Here's how the part is built. I have some questions about the finished solid (model axes, mm). Face numbers are marked on the shaded views. Round coordinates to 2 decimals unless told otherwise and drop trailing zeros. Write each loop counter-clockwise with the first axis right and the second up, starting at its lowest first coordinate (ties: lowest second). Pieces come first, ordered by that corner, then holes. Notation, with made-up numbers: (-35.5, -20.5) - (16.5, -20.5) arc R15 ccw to (16.5, -16.5) - close; hole circle Ø6 at (21, 73.5). An arc over 180 degrees is marked (long way). One line per item, written item: value. Start each with the question number.
Item 1: Imagine slicing it at B-B, the plane y = -0.85. Please give me the cut outline in (x, z), then the cut area to 3 significant figures.
Item 2: Imagine slicing it at A-A, the plane z = -12. Please give me the cut outline in (x, y), then the cut area to 3 significant figures.
Item 3: If I drill on line 1 (X direction, y = -0.3, z = -4); line 2 (X direction, y = -2.65, z = 11), over which ranges is the centre line in solid material (lowest first)?
Item 4: Thinking about a two-plate mould opening in Y: for the marked faces 1 and 2, which applies, released by +Y, released by -Y, zero draft, split by the parting line, or undercut?
Item 5: Imagine slicing it at C-C, the plane x = -15. Please give me the cut outline in (y, z), then the cut area to 3 significant figures.
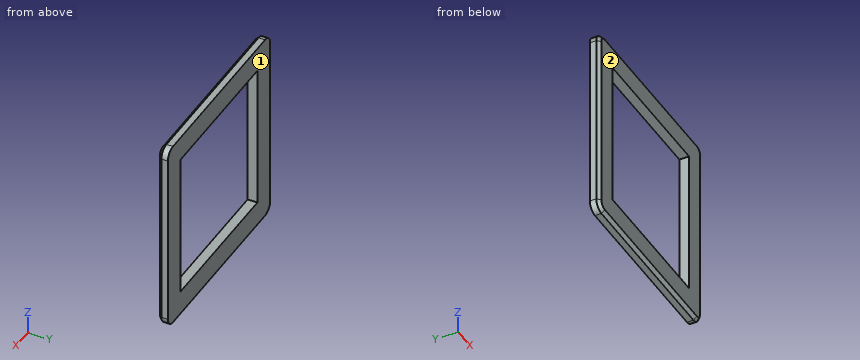
```python
from build123d import *

# Parameters (mm, degrees)
F0_W     = 45
F0_H     = 45
F1_DEPTH = 3
F2_SIZE  = 1


with BuildPart() as f1:
    # F0 (on Front) → F1 (new body)
    with BuildSketch(Plane.XZ):
        with BuildLine():
            Line((27, 30), (-27, 30))
            ThreePointArc((-27, 30), (-29.12132, 29.12132), (-30, 27))
            Line((-30, 27), (-30, -27))
            ThreePointArc((-30, -27), (-29.12132, -29.12132), (-27, -30))
            Line((-27, -30), (27, -30))
            ThreePointArc((27, -30), (29.12132, -29.12132), (30, -27))
            Line((30, -27), (30, 27))
            ThreePointArc((30, 27), (29.12132, 29.12132), (27, 30))
        make_face()
        Rectangle(F0_W, F0_H, mode=Mode.SUBTRACT)
    extrude(amount=F1_DEPTH)

    # F2
    f2_edges = [f1.edges().sort_by_distance(p)[0] for p in [
        (-30, -3, 0),
        (0, -3, 30),
        (30, -3, 0),
        (0, -3, -30),
    ]]
    chamfer(f2_edges, length=F2_SIZE)


solid = f1.part
```
Values follow:
1. outline: (-30, -27) arc R3 ccw to (-27, -30) - (27, -30) arc R3 ccw to (30, -27) - (30, 27) arc R3 ccw to (27, 30) - (-27, 30) arc R3 ccw to (-30, 27) - close; hole (-22.5, -22.5) - (22.5, -22.5) - (22.5, 22.5) - (-22.5, 22.5) - close
1. area: 1,570 mm^2
2. outline: (-30, -2) - (-29, -3) - (-22.5, -3) - (-22.5, 0) - (-30, 0) - close; (22.5, -3) - (29, -3) - (30, -2) - (30, 0) - (22.5, 0) - close
2. area: 44.0 mm^2
3. line 1: x = -30 to -22.5, 22.5 to 30
3. line 2: x = -29.35 to -22.5, 22.5 to 29.35
4. face 1: released by +Y
4. face 2: released by -Y
5. outline: (-3, -29) - (-2, -30) - (0, -30) - (0, -22.5) - (-3, -22.5) - close; (-3, 22.5) - (0, 22.5) - (0, 30) - (-2, 30) - (-3, 29) - close
5. area: 44.0 mm^2
